Geometry check sheet. Reference: the model listing, model coordinates, mm. Face numbers are marked on the shaded views. Coordinates: 2 decimals unless noted, no trailing zeros. Write each loop counter-clockwise with the first axis right and the second up, starting at its lowest first coordinate (ties: lowest second). Pieces come first, ordered by that corner, then holes. Notation, with made-up numbers: M -37.5,29 L -29.5,29 A21 cw -29.5,36 Z; hole C 57,39 d7. An arc over 180 degrees is marked long. Write each question's results on one line, items separated by ' | '.
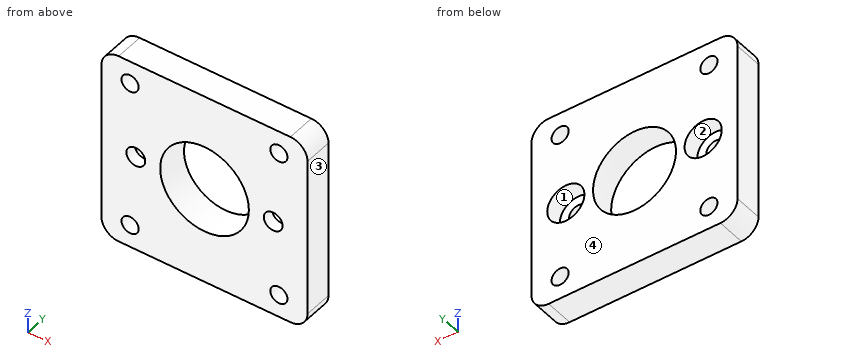
```python
from build123d import *

# Parameters (mm, degrees)
F0_W           = 36
F0_H           = 34
F0_R           = 1.5
F0_R_2         = 7.25
F1_DEPTH       = 5
F2_R           = 3
F3_SIZE2       = 4.99999
F3_SIZE        = 0.49999
F4_D           = 3.3
F4_CBORE_D     = 6.5
F4_CBORE_DEPTH = 3


# Not quite as in the source:
# - a fillet or chamfer is up to 0.001 mm smaller than in the source, because OpenCascade refuses the exact size


with BuildPart() as f1:
    # F0 (on Front) → F1 (new body)
    with BuildSketch(Plane.XZ):
        Rectangle(F0_W, F0_H)
        with Locations((-13, -13)):
            Circle(F0_R, mode=Mode.SUBTRACT)
        with Locations((13, -13)):
            Circle(F0_R, mode=Mode.SUBTRACT)
        with Locations((-13, 13)):
            Circle(F0_R, mode=Mode.SUBTRACT)
        Circle(F0_R_2, mode=Mode.SUBTRACT)
        with Locations((13, 13)):
            Circle(F0_R, mode=Mode.SUBTRACT)
    extrude(amount=F1_DEPTH)

    # F2
    f2_edges = [f1.edges().sort_by_distance(p)[0] for p in [
        (-18, -2.5, 17),
        (18, -2.5, 17),
        (18, -2.5, -17),
        (-18, -2.5, -17),
    ]]
    fillet(f2_edges, radius=F2_R)

    # F3 (size 0.5 and 5 in the source; OpenCascade refuses exactly that, so slightly less here)
    f3_edges = [f1.edges().sort_by_distance(p)[0] for p in [
        (-7.25, -5, 0),
    ]]
    f3_side = f1.faces().sort_by_distance((0, -5, -16.504823))[0]
    chamfer(f3_edges, length=F3_SIZE, length2=F3_SIZE2, reference=f3_side)

    # F4 (through all)
    with Locations(Plane(origin=(0, 0, 0), x_dir=(1, 0, 0), z_dir=(0, 1, 0))):
        with Locations((12, 0), (-12, 0)):
            CounterBoreHole(F4_D / 2, F4_CBORE_D / 2, F4_CBORE_DEPTH)


solid = f1.part
```
Q1. Sectioned sample at C-C on y = -2.2. Record the cut outline in (x, z).
Geometry check:
outline: M -18,-14 A3 ccw -15,-17 L 15,-17 A3 ccw 18,-14 L 18,14 A3 ccw 15,17 L -15,17 A3 ccw -18,14 Z; hole C -12,0 d6.5; hole C -13,-13 d3; hole C -13,13 d3; hole C 0,0 d14.94; hole C 12,0 d6.5; hole C 13,-13 d3; hole C 13,13 d3
Q2. Scan lines: probe 1 along X at (y, z) = (-0.8, 2); probe 2 along Z at (x, y) = (13, -2.7); probe 3 along X at (y, z) = (-0.85, 1.5). Record each from-to range of solid material in increasing order.
Geometry check:
probe 1: x = -18 to -14.56, -9.44 to -7.05, 7.05 to 9.44, 14.56 to 18 | probe 2: z = -17 to -14.5, -11.5 to -3.09, 3.09 to 11.5, 14.5 to 17 | probe 3: x = -18 to -14.88, -9.12 to -7.18, 7.18 to 9.12, 14.88 to 18
Q3. Depth check by flat-ended pin: P1, Ø5, axis at x = -12, z = 0, coming from the -Y side; P2, Ø3, axis at x = 12, z = 0, coming from the +Y side; P3, Ø2, axis at x = 10.5, z = 1.5, coming from the +Y side. Enter the tip coordinate at first touch or a pass-through.
Geometry check:
P1: stops at y = -5 | P2: passes through | P3: stops at y = -3
Q4. Mould release check, pull along X, two halves, no side actions. Record for the marked faces 1, 2, 3 and 4: pulls with the +X half, pulls with the -X half, needs draft (parallel to the pull), parting line crosses it, or undercut.
Geometry check:
face 1: undercut | face 2: undercut | face 3: pulls with the +X half | face 4: needs draft
Q5. Sectioned sample at A-A on z = 0. Give the number of separate pieces and of enclosed holes in the cut face, and give its area (3 significant figures).
Geometry check:
separate pieces: 4 | enclosed holes: 0 | area: 52.8 mm2
Q6. Sectioned sample at D-D on x = 12. Record the cut outline in (y, z), and give its area (3 significant figures).
Geometry check:
outline: M -5,-17 L 0,-17 L 0,-14.12 L -5,-14.12 Z; M -5,-11.88 L 0,-11.88 L 0,-3.25 L -3,-3.25 L -3,-1.65 L -5,-1.65 Z; M -5,1.65 L -3,1.65 L -3,3.25 L 0,3.25 L 0,11.88 L -5,11.88 Z; M -5,14.12 L 0,14.12 L 0,17 L -5,17 Z | area: 122 mm2
Q7. Sectioned sample at B-B on z = 13. Record the cut outline in (x, y).
Geometry check:
outline: M -18,-5 L -14.5,-5 L -14.5,0 L -18,0 Z; M -11.5,-5 L 11.5,-5 L 11.5,0 L -11.5,0 Z; M 14.5,-5 L 18,-5 L 18,0 L 14.5,0 Z
